from build123d import *

# Parameters (mm, degrees)
F0_W     = 100
F0_H     = 60
F1_DEPTH = 25
F2_R     = 7
F3_T     = -1


with BuildPart() as f1:
    # F0 (on Top) → F1 (new body)
    with BuildSketch(Plane.XY):
        Rectangle(F0_W, F0_H)
    extrude(amount=F1_DEPTH)

    # F2
    f2_edges = [f1.edges().sort_by_distance(p)[0] for p in [
        (0, -30, 25),
        (-50, 0, 25),
        (-50, -30, 12.5),
        (-50, 30, 12.5),
        (0, 30, 25),
        (50, 30, 12.5),
        (50, 0, 25),
        (50, -30, 12.5),
    ]]
    fillet(f2_edges, radius=F2_R)

    # F3
    f3_openings = [f1.faces().sort_by_distance(p)[0] for p in [
        (0, 0, 0),
    ]]
    offset(amount=F3_T, openings=f3_openings)


solid = f1.part
Here's how the part is built. I have some questions about the finished solid (model axes, mm). A direction names the side the tool comes from. Coordinates: 2 decimals unless noted, no trailing zeros. Write each loop counter-clockwise with the first axis right and the second up, starting at its lowest first coordinate (ties: lowest second). Pieces come first, ordered by that corner, then holes.
Item 1: If I drill on line 1 (Y direction, x = 14, z = 2.5); line 2 (X direction, y = 12, z = 17.25); line 3 (Z direction, x = 32.5, y = 5.5), over which ranges is the centre line in solid material (lowest first)?
Item 2: If we mould it in two halves opening along Y, with no side actions, what happens to faces 1 (the flat face through (50, 0, 9)), 2 (the cylindrical face through (47.289, 27.196, 9.126)), 3 (the flat face through (-1, 30, 9))? For each: +Y half, -Y half, draft (parallel to the pull), parting line (faces both ways), or undercut.
Item 3: On a 3-axis mill with a long thin cutter (end or side, diameter ignored), from which of +Z, -Z, +X, -X, +Y, -Y can I reach the whole of each face in a straight line? I mean faces 4 (the cylindrical face through (0.6, 28, 22.9)), 5 (the flat face through (-1, -29, 9)). Say none if no direction works.
Item 4: I want a section at B-B on y = -4.5. Write out the boundary of the cut face in (x, z), and give its area (3 significant figures).
Item 5: I want a section at A-A on z = 2.25. Write out the boundary of the cut face in (x, y).
Item 6: Will these pins go through, and if not, where does the flat tip stop? pin 1 (1.5 mm diameter, centred on y = -12.5, z = 19.5, fed in from -X); pin 2 (6 mm diameter, centred on x = 19.5, z = 20, fed in from -Y); pin 3 (4 mm diameter, centred on x = -10, z = 22, fed in from +Y).
Item 7: I want a section at C-C on x = -0.5. Write out the boundary of the cut face in (y, z).
Findings below:
1. line 1: y = -30 to -29, 29 to 30
1. line 2: x = -50 to -49, 49 to 50
1. line 3: z = 24 to 25
2. face 1: draft
2. face 2: undercut
2. face 3: +Y half
3. face 4: +Z, +X, -X, +Y
3. face 5: -Z
4. outline: (-50, 0) - (-49, 0) - (-49, 18) arc R6 cw to (-43, 24) - (43, 24) arc R6 cw to (49, 18) - (49, 0) - (50, 0) - (50, 18) arc R7 ccw to (43, 25) - (-43, 25) arc R7 ccw to (-50, 18) - close
4. area: 142 mm2
5. outline: (-50, -23) arc R7 ccw to (-43, -30) - (43, -30) arc R7 ccw to (50, -23) - (50, 23) arc R7 ccw to (43, 30) - (-43, 30) arc R7 ccw to (-50, 23) - close; hole (-49, -23) arc R6 ccw to (-43, -29) - (43, -29) arc R6 ccw to (49, -23) - (49, 23) arc R6 ccw to (43, 29) - (-43, 29) arc R6 ccw to (-49, 23) - close
6. pin 1: stops at x = -49.96
6. pin 2: stops at y = -30
6. pin 3: stops at y = 29.71
7. outline: (-30, 0) - (-29, 0) - (-29, 18) arc R6 cw to (-23, 24) - (23, 24) arc R6 cw to (29, 18) - (29, 0) - (30, 0) - (30, 18) arc R7 ccw to (23, 25) - (-23, 25) arc R7 ccw to (-30, 18) - close
